Autodesk Inventor part; units mm, degrees
ref_plane "YZ Plane" through (0, 0, 0) normal (1, 0, 0) x (0, 1, 0)
ref_plane "XZ Plane" through (0, 0, 0) normal (0, 1, 0) x (-1, 0, 0)
ref_plane "XY Plane" through (0, 0, 0) normal (0, 0, 1) x (1, 0, 0)
sketch "Sketch1" plane through (0, 0, 0) normal (0, 0, 1) x (1, 0, 0)
  circle A0 centre (0, 0) radius 14
  dimension "d0" = 28
extrude "Extrusion1" add sketch "Sketch1" along normal blind 41.5
sketch "Sketch2" plane through (0, 0, 41.5) normal (0, 0, 1) x (1, 0, 0)
  line L0 (-8.3964, 10.25) -> (8.3964, 10.25)
  line L1 (-8.3964, -10.25) -> (8.3964, -10.25)
  line L2 (-19.6, 0) -> (19.6, 0)
  arc A0 (8.3964, -10.25) -> (8.3964, 10.25) centre (0, 0) ccw
  arc A1 (-8.3964, 10.25) -> (-8.3964, -10.25) centre (0, 0) ccw
  dimension "d4" = 10.25
  dimension "d5" = 10.25
extrude "Extrusion2" add sketch "Sketch2" along normal blind 1
sketch "Sketch3" plane through (0, 0, 42.5) normal (0, 0, 1) x (1, 0, 0)
  circle A0 centre (0, 0) radius 5
  circle A1 centre (0, 0) radius 4.5
  dimension "d8" = 10
  dimension "d9" = 9
extrude "Extrusion3" add sketch "Sketch3" along normal blind 1.5
sketch "Sketch4" plane through (0, 0, 42.5) normal (0, 0, 1) x (1, 0, 0)
  circle A0 centre (0, 0) radius 4.5
  dimension "d12" = 9
extrude "Extrusion4" add sketch "Sketch4" along normal blind 1
sketch "Sketch5" plane through (0, 0, 43.5) normal (0, 0, 1) x (1, 0, 0)
  circle A0 centre (0, 0) radius 1.15
  dimension "d15" = 2.3
extrude "Extrusion5" add sketch "Sketch5" along normal blind 3
properties part number "E600T_RC390_motor_front"
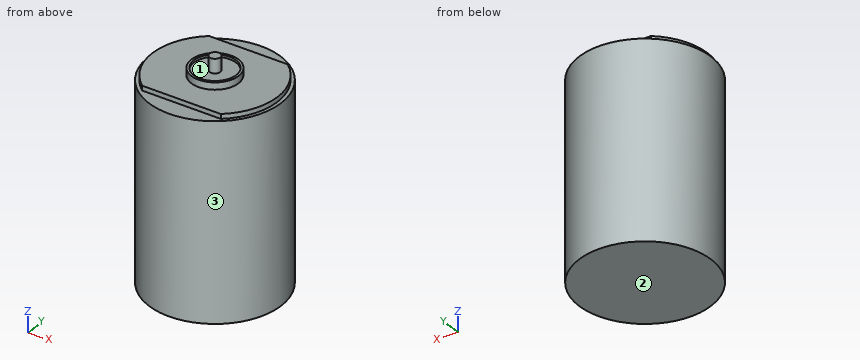
The listing builds one solid part. Answer for the finished solid, in the listing's coordinates (mm). Face numbers are marked on the shaded views. Give positions to 0.01 mm unless a question says otherwise; leave off trailing zeros. Loops run counter-clockwise (first coordinate to the right, second up) from the corner with the lowest first, then second, coordinate; pieces in that order, holes last. Notation, with made-up numbers: M -23,17.25 L 11,17.25 A11 ccw 11,22.25 Z; hole C -20.5,19.25 d10. An arc over 180 degrees is marked long. One line per item, written item: value.
1. Section D-D on x = 7.5 is taken. Determine the outline of the cut face in (y, z).
Found:
outline: M -11.82,0 L 11.82,0 L 11.82,41.5 L 10.25,41.5 L 10.25,42.5 L -10.25,42.5 L -10.25,41.5 L -11.82,41.5 Z
2. Find the intervals of material crossed by probe 1 along Y at (x, z) = (0, 43.85); probe 2 along Z at (x, y) = (-10.5, 6.25); probe 3 along Z at (x, y) = (5, 11.25), in increasing order.
Found:
probe 1: -5 to -4.5, -1.15 to 1.15, 4.5 to 5
probe 2: 0 to 42.5
probe 3: 0 to 41.5
3. Each of these flat-tipped pins is pushed along its axis until it touches: P1, Ø5, axis at x = 3, z = 15, coming from the +Y side; P2, Ø10, axis at x = -7, z = 19, coming from the -Y side; P3, Ø4, axis at y = -6, z = 33, coming from the +X side. Where does it stop, or does it pass through?
Found:
P1: y = 13.99
P2: y = -13.86
P3: x = 13.42
4. Section A-A on x = 0 is taken. Determine the outline of the cut face in (y, z).
Found:
outline: M -14,0 L 14,0 L 14,41.5 L 10.25,41.5 L 10.25,42.5 L 5,42.5 L 5,44 L 4.5,44 L 4.5,43.5 L 1.15,43.5 L 1.15,46.5 L -1.15,46.5 L -1.15,43.5 L -4.5,43.5 L -4.5,44 L -5,44 L -5,42.5 L -10.25,42.5 L -10.25,41.5 L -14,41.5 Z
5. Section B-B on y = 0 is taken. Determine the outline of the cut face in (x, z), plus the area to 3 significant figures.
Found:
outline: M -14,0 L 14,0 L 14,41.5 L 13.25,41.5 L 13.25,42.5 L 5,42.5 L 5,44 L 4.5,44 L 4.5,43.5 L 1.15,43.5 L 1.15,46.5 L -1.15,46.5 L -1.15,43.5 L -4.5,43.5 L -4.5,44 L -5,44 L -5,42.5 L -13.25,42.5 L -13.25,41.5 L -14,41.5 Z
area: 1,210 mm^2
6. For a pull along Y with two mould halves and no side action, classify the marked faces 1, 2 and 3 as pulls with the +Y half, pulls with the -Y half, needs draft (parallel to the pull), parting line crosses it, or undercut.
Found:
face 1: undercut
face 2: needs draft
face 3: parting line crosses it
7. Section C-C on z = 15.5 is taken. Determine the outline of the cut face in (x, y).
Found:
outline: C 0,0 d28
